```python
from build123d import *

# Parameters (mm, degrees)
SKETCH_1_W          = 28
SKETCH_1_H          = 20.3
SKETCH_1_R          = 1.5
EXTRUDE_1_DEPTH     = 5
SKETCH_2_W          = 28
SKETCH_2_H          = 6
SKETCH_2_H_2        = 4
EXTRUDE_2_DEPTH     = 10
SKETCH_3_W          = 28
SKETCH_3_H          = 6
EXTRUDE_3_DEPTH     = 5
FILLET_1_R          = 3
FILLET_2_R          = 1
SKETCH_4_R          = 1.5
CUT_EXTRUDE_1_DEPTH = 27.11173108


with BuildPart() as part:
    # 草图1 → 凸台-拉伸1 (new body)
    with BuildSketch(Plane.XY):
        Rectangle(SKETCH_1_W, SKETCH_1_H)
        with Locations((-5, 7.5)):
            Circle(SKETCH_1_R, mode=Mode.SUBTRACT)
        with Locations((5, 7.5)):
            Circle(SKETCH_1_R, mode=Mode.SUBTRACT)
        with Locations((5, -7.5)):
            Circle(SKETCH_1_R, mode=Mode.SUBTRACT)
        with Locations((-5, -7.5)):
            Circle(SKETCH_1_R, mode=Mode.SUBTRACT)
    extrude(amount=EXTRUDE_1_DEPTH)

    # 草图2 → 凸台-拉伸2 (add)
    with BuildSketch(Plane.XY.offset(5)):
        with Locations((0, 13.15)):
            Rectangle(SKETCH_2_W, SKETCH_2_H)
        with Locations((0, -12.15)):
            Rectangle(SKETCH_2_W, SKETCH_2_H_2)
    extrude(amount=-EXTRUDE_2_DEPTH)

    # 草图3 → 凸台-拉伸3 (add)
    with BuildSketch(Plane(origin=(0, 0, -5), x_dir=(-1, 0, 0), z_dir=(0, 0, -1))):
        with Locations((0, 13.15)):
            Rectangle(SKETCH_3_W, SKETCH_3_H)
    extrude(amount=EXTRUDE_3_DEPTH)

    # 圆角1
    fillet_1_edges = [part.edges().sort_by_distance(p)[0] for p in [
        (14, 16.15, -2.5),
        (0, -14.15, 5),
    ]]
    fillet(fillet_1_edges, radius=FILLET_1_R)

    # 圆角2
    fillet_2_edges = [part.edges().sort_by_distance(p)[0] for p in [
        (-14, 2.5, 5),
        (-14, 16.15, -2.5),
        (0, -14.15, -5),
        (-14, -14.15, -1.5),
        (-14, -13.271320344, 4.121320344),
    ]]
    fillet(fillet_2_edges, radius=FILLET_2_R)

    # 草图4 → 切除-拉伸1 (cut, through all)
    with BuildSketch(Plane.XY.offset(5)):
        with Locations((-9, 13.15)):
            Circle(SKETCH_4_R)
        with Locations((9, 13.15)):
            Circle(SKETCH_4_R)
    extrude(amount=-CUT_EXTRUDE_1_DEPTH, mode=Mode.SUBTRACT)


solid = part.part
```
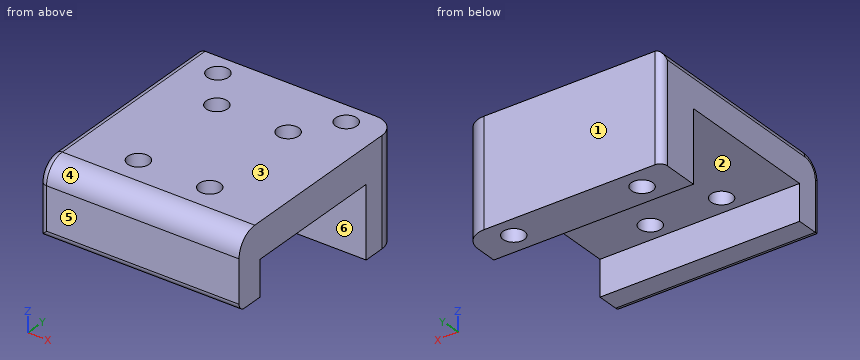
Geometry check sheet. Reference: the model listing, model coordinates, mm. Face numbers are marked on the shaded views. A direction names the side the tool comes from. Coordinates: 2 decimals unless noted, no trailing zeros. Write each loop counter-clockwise with the first axis right and the second up, starting at its lowest first coordinate (ties: lowest second). Pieces come first, ordered by that corner, then holes. Notation, with made-up numbers: M 15,54 L 20,54 A15 ccw 20,80 Z; hole C -29,-34.5 d2. An arc over 180 degrees is marked long. One line per item, written item: value. Start each with the question number.
(1) Sectioned sample at B-B, the plane x = 5. Enter the section's corners in (y, z), and give its area (3 significant figures).
(2) Scan lines: line 1 along Y through (x, z) = (-5, 1.4); line 2 along Y through (x, z) = (-1.5, -0.5); line 3 along Y through (x, z) = (5, 3.95). Record each from-to range of solid material in increasing order. Write a range as [from, to].
(3) Depth check by flat-ended pin: pin 1 (3.5 mm diameter, centred on x = 0, y = -11.5, fed in from -Z); pin 2 (5 mm diameter, centred on x = 5, y = -7.5, fed in from -Z). Enter the tip coordinate at first touch or a pass-through.
(4) Sectioned sample at A-A, the plane z = -1.75. Enter the section's corners in (x, y), and give its area (3 significant figures).
(5) Sectioned sample at C-C, the plane y = -7.5. Enter the section's corners in (x, z), and give its area (3 significant figures).
(6) Release check for a two-part mould opening along Y. For the marked faces 1, 2, 3 and 4 record: released by +Y, released by -Y, zero draft, split by the parting line, or undercut.
(7) Tool access check on the marked faces 5 and 6. Record the directions out of +Z, -Z, +X, -X, +Y, -Y that give a thin tool (end or side, any length) a straight path to the whole face; none if there is none.
(8) Sectioned sample at D-D, the plane x = 9. Enter the section's corners in (y, z).
Filled sheet:
1. outline: M -14.15,-4 A1 ccw -13.15,-5 L -10.15,-5 L -10.15,0 L -9,0 L -9,5 L -11.15,5 A3 ccw -14.15,2 Z; M -6,0 L 6,0 L 6,5 L -6,5 Z; M 9,0 L 10.15,0 L 10.15,-10 L 16.15,-10 L 16.15,5 L 9,5 Z
1. area: 199 mm²
2. line 1: [-14.15, -9], [-6, 6], [9, 16.15]
2. line 2: [-14.15, -10.15], [10.15, 16.15]
2. line 3: [-13.43, -9], [-6, 6], [9, 16.15]
3. pin 1: z = -5
3. pin 2: z = 0
4. outline: M -14,-13.15 A1 ccw -13,-14.15 L 14,-14.15 L 14,-10.15 L -14,-10.15 Z; M -14,10.15 L 14,10.15 L 14,13.15 A3 ccw 11,16.15 L -13,16.15 A1 ccw -14,15.15 Z; hole C -9,13.15 d3; hole C 9,13.15 d3
4. area: 264 mm²
5. outline: M -14,0 L -6.5,0 L -6.5,5 L -13,5 A1 ccw -14,4 Z; M -3.5,0 L 3.5,0 L 3.5,5 L -3.5,5 Z; M 6.5,0 L 14,0 L 14,5 L 6.5,5 Z
5. area: 110 mm²
6. face 1: released by +Y
6. face 2: undercut
6. face 3: zero draft
6. face 4: released by -Y
7. face 5: +Z, -Z, +X, -X, -Y
7. face 6: -Z, +X, -X
8. outline: M -14.15,-4 A1 ccw -13.15,-5 L -10.15,-5 L -10.15,0 L 10.15,0 L 10.15,-10 L 11.65,-10 L 11.65,5 L -11.15,5 A3 ccw -14.15,2 Z; M 14.65,-10 L 16.15,-10 L 16.15,5 L 14.65,5 Z
